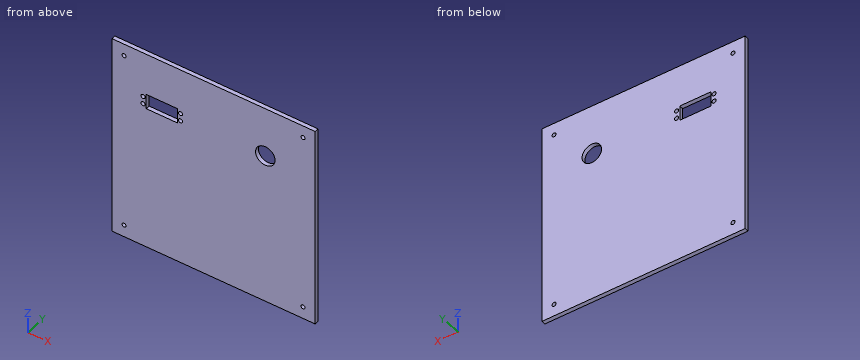
from build123d import *

# Parameters (mm, degrees)
SCHIZZO1_W                   = 250
SCHIZZO1_H                   = 250
SCHIZZO1_R                   = 2.5
SCHIZZO1_R_2                 = 12
SCHIZZO1_R_3                 = 2.54
SCHIZZO1_W_2                 = 38.23
SCHIZZO1_H_2                 = 18.54
ESTRUSIONE_ESTRUSIONE1_DEPTH = 5


with BuildPart() as part:
    # Schizzo1 → Estrusione-Estrusione1 (new body)
    with BuildSketch(Plane(origin=(0, 0, 0), x_dir=(1, 0, 0), z_dir=(0, 1, 0))):
        Rectangle(SCHIZZO1_W, SCHIZZO1_H)
        with Locations(Location((-110, 110, 0), (0, 0, 270))):
            Circle(SCHIZZO1_R, mode=Mode.SUBTRACT)
        with Locations(Location((110, 110, 0), (0, 0, 270))):
            Circle(SCHIZZO1_R, mode=Mode.SUBTRACT)
        with Locations(Location((-110, -110, 0), (0, 0, 270))):
            Circle(SCHIZZO1_R, mode=Mode.SUBTRACT)
        with Locations(Location((110, -110, 0), (0, 0, 270))):
            Circle(SCHIZZO1_R, mode=Mode.SUBTRACT)
        with Locations(Location((63.639610307, -63.639610307, 0), (0, 0, 270))):
            Circle(SCHIZZO1_R_2, mode=Mode.SUBTRACT)
        with Locations(Location((-86.655104778, -58.939610307, 0), (0, 0, 270))):
            Circle(SCHIZZO1_R_3, mode=Mode.SUBTRACT)
        with Locations(Location((-86.655104778, -68.337610307, 0), (0, 0, 270))):
            Circle(SCHIZZO1_R_3, mode=Mode.SUBTRACT)
        with Locations(Location((-40.621115836, -68.337610307, 0), (0, 0, 270))):
            Circle(SCHIZZO1_R_3, mode=Mode.SUBTRACT)
        with Locations(Location((-40.621115836, -58.939610307, 0), (0, 0, 270))):
            Circle(SCHIZZO1_R_3, mode=Mode.SUBTRACT)
        with Locations((-63.639610307, -63.639610307)):
            Rectangle(SCHIZZO1_W_2, SCHIZZO1_H_2, mode=Mode.SUBTRACT)
    extrude(amount=ESTRUSIONE_ESTRUSIONE1_DEPTH)


solid = part.part
Input: part model. Units: mm. Frame: model coordinates. Coordinates: 2 decimals unless noted, no trailing zeros. Answer as a JSON object with one key per item and string values. Group by question number.
(1) Section A-A on y = 3.4. Give the number of separate pieces and of enclosed holes in the cut face, plus the area to 3 significant figures.
(2) Ray query, line 1 along X through (y, z) = (2.45, -110); line 2 along Z through (x, y) = (-75, 3.45). Return the intervals inside material, ascending. Write a range as [from, to].
(3) Contact query for a flat-ended pin moving along its axis: P1, Ø14.5, axis at x = 63.64, z = 63.64, coming from the -Y side. Output: stop coordinate, or through.
Result set:
{
 "1": {"separate pieces": "1", "enclosed holes": "10", "area": "61,200 mm2"},
 "2": {"line 1": "x = [-125, -112.5], [-107.5, 107.5], [112.5, 125]", "line 2": "z = [-125, 54.37], [72.91, 125]"},
 "3": {"P1": "passes through"}
}
